Input: part model. Units: mm. Frame: model coordinates. A direction names the side the tool comes from. Give positions to 0.01 mm unless a question says otherwise; leave off trailing zeros. Loops run counter-clockwise (first coordinate to the right, second up) from the corner with the lowest first, then second, coordinate; pieces in that order, holes last. Notation, with made-up numbers: (62.25, 35.25) -> (67.25, 35.25) arc R20 cw to (67.25, 66.25) -> close; hole circle Ø9 at (-17.75, -30.75). An arc over 180 degrees is marked (long way). Answer as a JSON object with one key per item and string values.
Autodesk Inventor part; units mm, degrees
ref_plane "YZ Plane" through (0, 0, 0) normal (1, 0, 0) x (0, 1, 0)
ref_plane "XZ Plane" through (0, 0, 0) normal (0, 1, 0) x (-1, 0, 0)
ref_plane "XY Plane" through (0, 0, 0) normal (0, 0, 1) x (1, 0, 0)
sketch "Sketch1" plane through (0, 0, 0) normal (0, 1, 0) x (-1, 0, 0)
  circle A0 centre (0, 0) radius 2
  arc A1 (2.1, -2.1424) -> (-2.1, -2.1424) centre (0, 0) ccw
  circle A2 centre (0, -25.6944) radius 2
  arc A3 (-2.1, -23.5519) -> (2.1, -23.5519) centre (0, -25.6944) ccw
  line L0 (1.5, -3.5707) -> (1.5, -22.1236)
  line L1 (-1.5, -3.5707) -> (-1.5, -22.1236)
  line L2 (0, 0) -> (0, -25.6944) construction
  arc A4 (2.1, -2.1424) -> (1.5, -3.5707) centre (3.5, -3.5707) ccw
  arc A5 (-1.5, -3.5707) -> (-2.1, -2.1424) centre (-3.5, -3.5707) ccw
  arc A6 (-2.1, -23.5519) -> (-1.5, -22.1236) centre (-3.5, -22.1236) ccw
  arc A7 (1.5, -22.1236) -> (2.1, -23.5519) centre (3.5, -22.1236) ccw
  point P0 (1.5, -2.5981)
  point P1 (-1.5, -23.0963)
  point P2 (-1.5, -2.5981)
  point P3 (1.5, -23.0963)
  dimension "d0" = 4
  dimension "d1" = 6
  dimension "d2" = 25.6944
  dimension "d3" = 4
  dimension "d4" = 6
  dimension "d5" = 3
  dimension "d6" = 2
extrude "Extrusion1" add sketch "Sketch1" along normal blind 2
equation "\"d3\" = d0"
equation "\"d4\" = d1"
equation "\"length\" = 25.69436"
properties part number "dip_pip_tendon"
Q1. Section D-D, the plane z = -7. Return the cut outline in (x, y), then the cut area to 3 significant figures.
Evaluation:
{"outline": "(-1.5, 0) -> (1.5, 0) -> (1.5, 2) -> (-1.5, 2) -> close", "area": "6.00 mm2"}
Q2. Draft query along X for faces 4 (the cylindrical face through (0.26, 0.986, -27.677)), 5 (the cylindrical face through (0, 1, 2)), 6 (the cylindrical face through (-0.099, 0.986, -28.693)), 7 (the cylindrical face through (-1.65, 0.99, -2.81)). Return one class per face: +X half, -X half, draft (parallel to the pull), parting line (faces both ways), or undercut.
Evaluation:
{"face 4": "undercut", "face 5": "undercut", "face 6": "parting line", "face 7": "-X half"}
Q3. Section B-B, the plane z = 0. Return the cut outline in (x, y), then the cut area to 3 significant figures.
Evaluation:
{"outline": "(-3, 0) -> (-2, 0) -> (-2, 2) -> (-3, 2) -> close; (2, 0) -> (3, 0) -> (3, 2) -> (2, 2) -> close", "area": "4.00 mm2"}
Q4. Section C-C, the plane y = 0.65. Return the cut outline in (x, z).
Evaluation:
{"outline": "(-2.1, -23.55) arc R3 ccw (long way) to (2.1, -23.55) arc R2 cw to (1.5, -22.12) -> (1.5, -3.57) arc R2 cw to (2.1, -2.14) arc R3 ccw (long way) to (-2.1, -2.14) arc R2 cw to (-1.5, -3.57) -> (-1.5, -22.12) arc R2 cw to start; hole circle Ø4 at (0, -25.69); hole circle Ø4 at (0, 0)"}
Q5. Pin query (flat end, axial travel): pin 1 (0.6 mm diameter, centred on y = 1, z = -10, fed in from +X); pin 2 (3 mm diameter, centred on x = 2, z = -15.5, fed in from +Y); pin 3 (1 mm diameter, centred on y = 1, z = -24, fed in from -X). Return the tip coordinate at first contact, or that it passes through.
Evaluation:
{"pin 1": "stops at x = 1.5", "pin 2": "stops at y = 2", "pin 3": "stops at x = -2.75"}
Q6. Section A-A, the plane x = 0. Return the cut outline in (y, z).
Evaluation:
{"outline": "(0, -28.69) -> (2, -28.69) -> (2, -27.69) -> (0, -27.69) -> close; (0, -23.69) -> (2, -23.69) -> (2, -2) -> (0, -2) -> close; (0, 2) -> (2, 2) -> (2, 3) -> (0, 3) -> close"}
Q7. Ray query, line 1 along Z through (x, y) = (-0.25, 1.65); line 2 along Z through (x, y) = (-1.25, 1.3); line 3 along X through (y, z) = (1.4, -11.5). Return the intervals inside material, ascending.
Evaluation:
{"line 1": "z = -28.68 to -27.68, -23.71 to -1.98, 1.98 to 2.99", "line 2": "z = -28.42 to -27.26, -24.13 to -1.56, 1.56 to 2.73", "line 3": "x = -1.5 to 1.5"}
Q8. Access query for faces 1 (the cylindrical face through (1.652, 0.986, -22.888)), 2 (the cylindrical face through (0, 1, 3)), 3 (the flat face through (-1.5, 1, -13)). Directions: +Z, -Z, +X, -X, +Y, -Y. A direction counts if a zero-diameter tool reaches every point of the face in a straight line with its end or side. Return the directions, or none.
Evaluation:
{"face 1": "+X, +Y, -Y", "face 2": "+Y, -Y", "face 3": "-X, +Y, -Y"}
